Check sheet for the modelled part. Datum: model origin and axes. Units: mm. Round coordinates to 2 decimals unless told otherwise and drop trailing zeros. Order: outer loops, then holes, each group sorted by start corner. A loop starts at its lowest first (then second) coordinate and runs counter-clockwise, first axis right, second up.
Q1. Cross-section at A-A on z = 34. Record the cut outline in (x, y).
Q2. Cross-section at C-C on y = 507. Record the cut outline in (x, z), then the cut area to 4 significant figures.
Q3. Scan lines: probe 1 along Y at (x, z) = (-1010, 6); probe 2 along Y at (x, z) = (-700.5, 30); probe 3 along X at (y, z) = (70, 7). Record each from-to range of solid material in increasing order.
Q4. Cross-section at B-B on x = -73. Record the cut outline in (y, z), then the cut area to 4 significant figures.
Q5. Depth check by flat-ended pin: P1, Ø1.5, axis at y = 640, z = 16.5, coming from the +X side; P2, Ø1, axis at x = -924.5, y = 92, coming from the +Z side; P3, Ø1.8, axis at x = -1009.5, y = 69, coming from the -Z side. Enter the tip coordinate at first touch or a pass-through.
Q6. Mould release check, pull along Y, two halves, no side actions. Record for faces 1 (the flat face through (-548, 780, 20)), 2 (the flat face through (-547, 395, 25)), 3 (the flat face through (-548, 395, 0)), 4 (the flat face through (-548, 0, 20)): +Y half, -Y half, draft (parallel to the pull), parting line (faces both ways), or undercut.
from build123d import *

# Parameters (mm, degrees)
F0_W     = 1080
F0_H     = 780
F1_DEPTH = 40
F2_R     = 3
F3_DEPTH = 12
F4_W     = 990
F4_H     = 690
F5_DEPTH = 15


with BuildPart() as f1:
    # F0 (on Top) → F1 (new body)
    with BuildSketch(Plane.XY):
        with Locations((-540, 390)):
            Rectangle(F0_W, F0_H)
    extrude(amount=F1_DEPTH)

    # F2 (on face) → F3 (cut)
    with BuildSketch(Plane(origin=(0, 0, 0), x_dir=(1, 0, 0), z_dir=(0, 0, -1))):
        with Locations((-1010, -70)):
            Circle(F2_R)
    extrude(amount=-F3_DEPTH, mode=Mode.SUBTRACT)

    # F4 (on face) → F5 (cut)
    with BuildSketch(Plane.XY.offset(40)):
        with Locations((-540, 390)):
            Rectangle(F4_W, F4_H)
    extrude(amount=-F5_DEPTH, mode=Mode.SUBTRACT)


solid = f1.part
Results found:
1. outline: (-1080, 0) - (0, 0) - (0, 780) - (-1080, 780) - close; hole (-1035, 45) - (-45, 45) - (-45, 735) - (-1035, 735) - close
2. outline: (-1080, 0) - (0, 0) - (0, 40) - (-45, 40) - (-45, 25) - (-1035, 25) - (-1035, 40) - (-1080, 40) - close
2. area: 28,350 mm2
3. probe 1: y = 0 to 67, 73 to 780
3. probe 2: y = 0 to 45, 735 to 780
3. probe 3: x = -1080 to -1013, -1007 to 0
4. outline: (0, 0) - (780, 0) - (780, 40) - (735, 40) - (735, 25) - (45, 25) - (45, 40) - (0, 40) - close
4. area: 20,850 mm2
5. P1: stops at x = 0
5. P2: stops at z = 25
5. P3: stops at z = 12
6. face 1: +Y half
6. face 2: undercut
6. face 3: draft
6. face 4: -Y half
